```python
from build123d import *

# Parameters (mm, degrees)
F1_DEPTH = 50
F2_SIZE  = 4.99999
F3_R     = 4.25
F4_DEPTH = 25


# Not quite as in the source:
# - a fillet or chamfer is up to 0.001 mm smaller than in the source, because OpenCascade refuses the exact size


with BuildPart() as f1:
    # F0 (on Top) → F1 (new body)
    with BuildSketch(Plane.XY):
        Polygon((40, 23.61271578), (0, 23.61271578), (0, 18.61271578), (35, 18.61271578), (35, -16.38728422), (40, -16.38728422), align=None)
    extrude(amount=F1_DEPTH)

    # F2 (size 5 in the source; OpenCascade refuses exactly that, so slightly less here)
    f2_edges = [f1.edges().sort_by_distance(p)[0] for p in [
        (0, 18.612716, 25),
        (35, -16.387284, 25),
    ]]
    chamfer(f2_edges, length=F2_SIZE)

    # F3 (on face) → F4 (cut)
    with BuildSketch(Plane.YZ.offset(40)):
        with Locations((8.61271578, 25)):
            Circle(F3_R)
    extrude(amount=-F4_DEPTH, mode=Mode.SUBTRACT)


solid = f1.part
```
Geometry: final body of the model. Coordinates: model frame, mm. A direction names the side the tool comes from. Round coordinates to 2 decimals unless told otherwise and drop trailing zeros. Loops run counter-clockwise (first coordinate to the right, second up) from the corner with the lowest first, then second, coordinate; pieces in that order, holes last. Notation, with made-up numbers: (39, 25.25) -> (62, 25.25) arc R22 ccw to (62, 50.25) -> close; hole circle Ø9 at (40.5, -17.75). An arc over 180 degrees is marked (long way). Use one line per item in the form item = value. Start each with the question number.
1) Access query for faces 1 (the flat face through (20, 18.613, 25)), 2 (the flat face through (29, 20, 50)). Directions: +Z, -Z, +X, -X, +Y, -Y. A direction counts if a zero-diameter tool reaches every point of the face in a straight line with its end or side. Return the directions, or none.
2) First-contact query: P1, Ø15, axis at y = 7, z = 34, coming from the -X side; P2, Ø10, axis at x = 9, z = 36.5, coming from the -Y side. Flat tips, straight axial feed; report the tip coordinate or a pass-through.
3) Section C-C on y = 17. Output: boundary loops of the cut face in (x, z), then the cut area to 3 significant figures.
4) Section D-D on x = 28. Output: boundary loops of the cut face in (y, z).
5) Line query: L1, parallel to X at y = 13, z = 19.5; L2, parallel to Y at x = 5.5, z = 33; L3, parallel to Y at x = 35.5, z = 28.5. Output: solid intervals per line, ascending.
Response:
q1.face_1 = +Z, -Z, -X, -Y
q1.face_2 = +Z, +X, -X, +Y, -Y
q2.P1 = 35
q2.P2 = 18.61
q3.outline = (35, 0) -> (40, 0) -> (40, 50) -> (35, 50) -> close
q3.area = 250 mm^2
q4.outline = (18.61, 0) -> (23.61, 0) -> (23.61, 50) -> (18.61, 50) -> close
q5.L1 = 35 to 40
q5.L2 = 18.61 to 23.61
q5.L3 = -11.89 to 6.2, 11.02 to 23.61
